Can you work these out from the model? Positions are in its coordinate system, mm. Face numbers are marked on the shaded views. Round coordinates to 2 decimals unless told otherwise and drop trailing zeros. Loops run counter-clockwise (first coordinate to the right, second up) from the corner with the lowest first, then second, coordinate; pieces in that order, holes last. Notation, with made-up numbers: (87, -19.75) -> (98, -19.75) arc R23 cw to (98, 3.25) -> close; hole circle Ø2 at (49.25, -35). An arc over 180 degrees is marked (long way). Write each question's results on one line, items separated by ' | '.
from build123d import *

# Parameters (mm, degrees)
CROQUIS1_W              = 175
CROQUIS1_H              = 582
SALIENTE_EXTRUIR1_DEPTH = 35
CROQUIS2_W              = 105
CROQUIS2_H              = 582
CORTAR_EXTRUIR1_DEPTH   = 20
CROQUIS3_W              = 105
CROQUIS3_H              = 432
CORTAR_EXTRUIR2_DEPTH   = 305.527913335


with BuildPart() as part:
    # Croquis1 → Saliente-Extruir1 (new body)
    with BuildSketch(Plane(origin=(0, 0, 0), x_dir=(1, 0, 0), z_dir=(0, 1, 0))):
        Rectangle(CROQUIS1_W, CROQUIS1_H)
    extrude(amount=SALIENTE_EXTRUIR1_DEPTH)

    # Croquis2 → Cortar-Extruir1 (cut)
    with BuildSketch(Plane(origin=(0, 35, 0), x_dir=(1, 0, 0), z_dir=(0, 1, 0))):
        Rectangle(CROQUIS2_W, CROQUIS2_H)
    extrude(amount=-CORTAR_EXTRUIR1_DEPTH, mode=Mode.SUBTRACT)

    # Croquis3 → Cortar-Extruir2 (cut, through all)
    with BuildSketch(Plane(origin=(0, 15, 0), x_dir=(1, 0, 0), z_dir=(0, 1, 0))):
        Rectangle(CROQUIS3_W, CROQUIS3_H)
    extrude(amount=-CORTAR_EXTRUIR2_DEPTH, mode=Mode.SUBTRACT)


solid = part.part
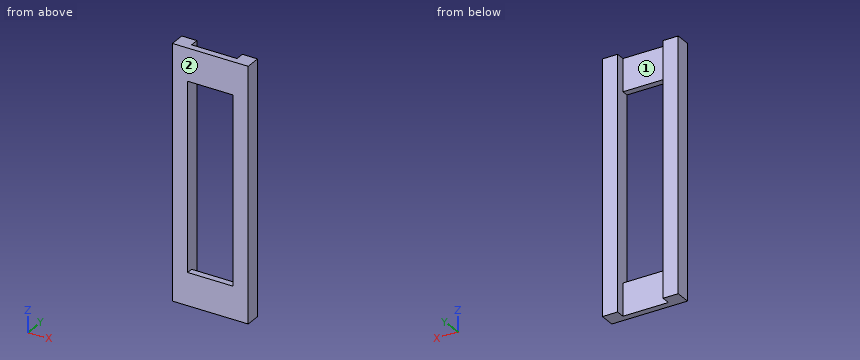
1. Will these pins go through, and if not, where does the flat tip stop? pin 1 (5 mm diameter, centred on x = 51, z = 171.5, fed in from +Y); pin 2 (22.5 mm diameter, centred on x = 13, z = -265, fed in from +Y).
Final values:
pin 1: y = 35 | pin 2: y = 15
2. If we section it at D-D (z = 247): List the corners of the cut face in (x, y) for me, then the cut area to 4 significant figures.
Final values:
outline: (-87.5, 0) -> (87.5, 0) -> (87.5, 35) -> (52.5, 35) -> (52.5, 15) -> (-52.5, 15) -> (-52.5, 35) -> (-87.5, 35) -> close | area: 4,025 mm2
3. Please list where these lines run through material, in increasing order: line 1 (X direction, y = 31.5, z = -212); line 2 (Z direction, x = 6.5, y = 13.5); line 3 (Y direction, x = -3.5, z = 258). Write a range as from..to.
Final values:
line 1: -87.5..-52.5, 52.5..87.5 | line 2: -291..-216, 216..291 | line 3: 0..15
4. If we section it at A-A (z = -26.5): List the corners of the cut face in (x, y) for me, then the cut area to 3 significant figures.
Final values:
outline: (-87.5, 0) -> (-52.5, 0) -> (-52.5, 35) -> (-87.5, 35) -> close; (52.5, 0) -> (87.5, 0) -> (87.5, 35) -> (52.5, 35) -> close | area: 2,450 mm2
5. If we section it at C-C (y = 7.5): List the corners of the cut face in (x, z) for me.
Final values:
outline: (-87.5, -291) -> (87.5, -291) -> (87.5, 291) -> (-87.5, 291) -> close; hole (-52.5, -216) -> (52.5, -216) -> (52.5, 216) -> (-52.5, 216) -> close
6. We'd pull the mould along X, two halves only. Please class the marked faces 1 and 2: pulls with the +X half, pulls with the -X half, needs draft (parallel to the pull), parting line crosses it, or undercut.
Final values:
face 1: undercut | face 2: needs draft
7. If we section it at B-B (x = -36): List the corners of the cut face in (y, z) for me.
Final values:
outline: (0, -291) -> (15, -291) -> (15, -216) -> (0, -216) -> close; (0, 216) -> (15, 216) -> (15, 291) -> (0, 291) -> close
